Part model, mm, in its own coordinate system. A direction names the side the tool comes from. Round coordinates to 2 decimals unless told otherwise and drop trailing zeros. Write each loop counter-clockwise with the first axis right and the second up, starting at its lowest first coordinate (ties: lowest second). Pieces come first, ordered by that corner, then holes. Notation, with made-up numbers: M 31.5,55 L 64.5,55 A23 ccw 64.5,82 Z; hole C 30,40 d8. An arc over 180 degrees is marked long. One line per question, with ' | ' between items. Start each with the question number.
1) Saw through at A-A (z = 0). List the corners of the cut face in (x, y).
2) Drop flat-ended pins along their axis: pin 1 Ø1 at (x, y) = (14, -39.5) entering from -Z; pin 2 Ø4 at (y, z) = (-22, -2.5) entering from -X; pin 3 Ø6 at (y, z) = (6.5, -3) entering from +X. Give the stop position or say it passes through.
3) Tool access for faces 3 (the face through (23.54, -32.19, -2.3)), 4 (the face through (-18, -65, 0)): list every direction of +Z, -Z, +X, -X, +Y, -Y with a clear straight run to the whole face (end or side of a thin tool).
4) Mould opens along X. For faces 1 (the face through (-23.54, -31.31, -2.3)), 2 (the face through (18, -65, 0)) say: pulls with the +X half, pulls with the -X half, needs draft (parallel to the pull), parting line crosses it, or undercut.
5) Wall check: probe 1 along X at (y, z) = (-8, -0.5); probe 2 along X at (y, z) = (-48, -1); probe 3 along Y at (x, z) = (-15, 4.25). Give the ranges that are in metal, low to high. Write a range as [from, to].
6) Saw through at B-B (y = -24.5). List the corners of the cut face in (x, z).
Autodesk Fusion 360 part; units mm, degrees
sketch "Sketch1" plane through (0, 0, 0) normal (0, 0, 1) x (1, 0, 0)
  circle A0 centre (0, 0) radius 18 construction
  line L0 (0, 0) -> (50, 0) construction
  line L1 (0, 0) -> (0, 50) construction
  line L2 (0, 0) -> (-50, 0) construction
  line L3 (0, 0) -> (0, -100) construction
  line L4 (-18, 0) -> (-18, -65)
  line L5 (18, 0) -> (18, -65)
  arc A1 (18, 0) -> (-18, 0) centre (0, 0) ccw
  dimension "d1" = 36
  dimension "d6" = 65
  dimension "d7" = 65
sketch "Sketch2" plane through (0, 0, 0) normal (0, 1, 0) x (1, 0, 0)
  circle A0 centre (18, 0) radius 6
  point P0 (18, 0)
  dimension "d8" = 12
sweep "Sweep1" add profiles "Sketch2" path "Sketch1" along L5 A1 L4 section 1
chamfer "Chamfer1" distance 1.5 angle 45 2 edges at (-12.406, -65, 2.1697) (12.406, -65, -2.1697)
thread "Thread1"
thread "Thread2"
Answer key:
1) outline: M -24,-63.5 L -22.5,-65 L -13.5,-65 L -12,-63.5 L -12,0 A12 cw 12,0 L 12,-63.5 L 13.5,-65 L 22.5,-65 L 24,-63.5 L 24,0 A24 ccw -24,0 Z
2) pin 1: stops at z = -4.87 | pin 2: stops at x = -23.98 | pin 3: stops at x = 23.53
3) face 3: -Y | face 4: +Z, -Z, +X, -X, -Y
4) face 1: undercut | face 2: needs draft
5) probe 1: x = [-23.98, -12.02], [12.02, 23.98] | probe 2: x = [-23.92, -12.08], [12.08, 23.92] | probe 3: y = [-64.3, 16.41]
6) outline: C -18,0 d12; C 18,0 d12
